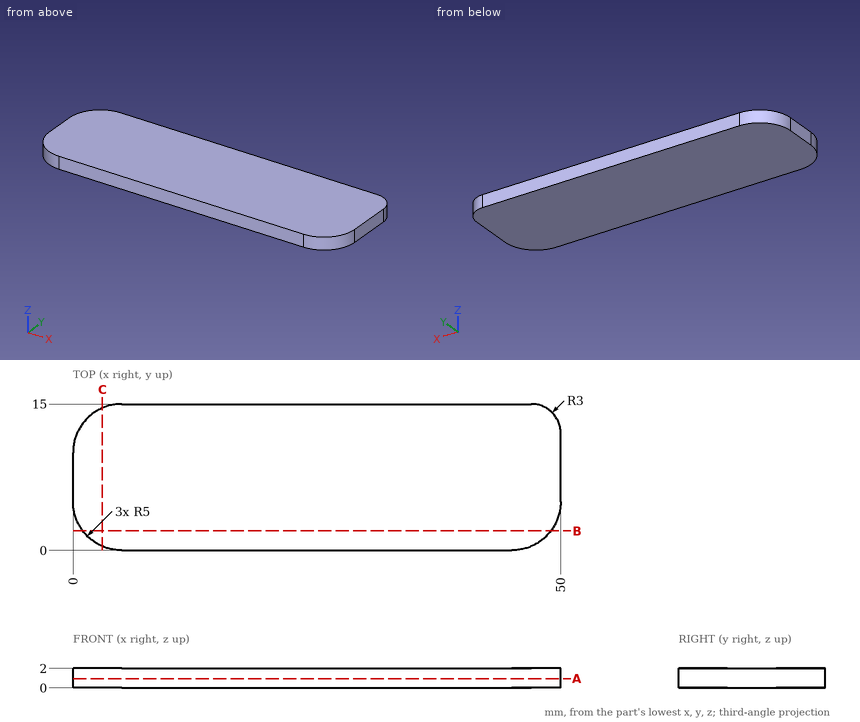
For this review, use the dimensioned drawing (mm, ordinates from the lowest corner) and the shaded views. Round coordinates to 2 decimals unless told otherwise and drop trailing zeros. Write each loop counter-clockwise with the first axis right and the second up, starting at its lowest first coordinate (ties: lowest second). Pieces come first, ordered by that corner, then holes. Notation, with made-up numbers: M -17,2 L -3,2 A36 cw -3,40 Z; hole C -13,33 d10. An arc over 180 degrees is marked long. Write item = value, one per line. Start each with the question number.
(1) We need section B-B (y = 2). Give the boundary of the cut face in (x, z), then the cut area to 3 significant figures.
(2) For line 1 along X through (y, z) = (10.25, 0.5); line 2 along X through (y, z) = (12.25, 1.25), list the stretches that pass through material, from the lowest coordinate up.
(3) We need section A-A (z = 0.95). Give the boundary of the cut face in (x, y), then the cut area to 3 significant figures.
(4) We need section C-C (x = 3). Give the boundary of the cut face in (y, z), then the cut area to 3 significant figures.
Results found:
q1.outline = M 1,0 L 49,0 L 49,2 L 1,2 Z
q1.area = 96.0 mm²
q2.line_1 = 0.01 to 50
q2.line_2 = 0.53 to 49.99
q3.outline = M 0,5 A5 ccw 5,0 L 45,0 A5 ccw 50,5 L 50,12 A3 ccw 47,15 L 5,15 A5 ccw 0,10 Z
q3.area = 732 mm²
q4.outline = M 0.42,0 L 14.58,0 L 14.58,2 L 0.42,2 Z
q4.area = 28.3 mm²
